Input: part model. Units: mm. Frame: model coordinates. A direction names the side the tool comes from. Coordinates: 2 decimals unless noted, no trailing zeros. Order: outer loops, then holes, each group sorted by start corner. A loop starts at its lowest first (then second) coordinate and runs counter-clockwise, first axis right, second up.
from build123d import *

# Parameters (mm, degrees)
SKETCH1_R           = 1.5
BOSS_EXTRUDE1_DEPTH = 10
BOSS_EXTRUDE2_DEPTH = 1.75
SKETCH3_R           = 3
CUT_EXTRUDE1_DEPTH  = 5


with BuildPart() as part:
    # Sketch1 → Boss-Extrude1 (new body)
    with BuildSketch(Plane(origin=(0, 0, 0), x_dir=(1, 0, 0), z_dir=(0, 1, 0))):
        with BuildLine():
            ThreePointArc((-43.97114317, 22.5), (-38.97114317, 17.5), (-33.97114317, 22.5))
            Line((-33.97114317, 22.5), (-33.97114317, 54.272052467))
            Line((-33.97114317, 54.272052467), (33.97114317, 54.272052467))
            Line((33.97114317, 54.272052467), (33.97114317, 22.5))
            ThreePointArc((33.97114317, 22.5), (38.97114317, 17.5), (43.97114317, 22.5))
            Line((43.97114317, 22.5), (43.97114317, 64.272052467))
            Line((43.97114317, 64.272052467), (-43.97114317, 64.272052467))
            Line((-43.97114317, 64.272052467), (-43.97114317, 22.5))
        make_face()
        with Locations(Location((-38.97114317, 22.5, 0), (0, 0, 270))):
            Circle(SKETCH1_R, mode=Mode.SUBTRACT)
        with Locations(Location((38.97114317, 22.5, 0), (0, 0, 270))):
            Circle(SKETCH1_R, mode=Mode.SUBTRACT)
        with Locations(Location((7.5, 59.272052467, 0), (0, 0, 270))):
            Circle(SKETCH1_R, mode=Mode.SUBTRACT)
        with Locations(Location((-7.5, 59.272052467, 0), (0, 0, 270))):
            Circle(SKETCH1_R, mode=Mode.SUBTRACT)
    extrude(amount=BOSS_EXTRUDE1_DEPTH)

    # Sketch2 → Boss-Extrude2 (add)
    # profile 1 of 2: a face of its own
    with BuildSketch(Plane.XZ):
        Polygon((-1.726497308, -59.272052467), (-4.613248654, -54.272052467), (-10.386751346, -54.272052467), (-13.273502692, -59.272052467), (-10.386751346, -64.272052467), (-4.613248654, -64.272052467), align=None)
        Polygon((-9.232050808, -56.272052467), (-5.767949192, -56.272052467), (-4.035898385, -59.272052467), (-5.767949192, -62.272052467), (-9.232050808, -62.272052467), (-10.964101615, -59.272052467), align=None, mode=Mode.SUBTRACT)
    # profile 2 of 2: a face of its own
    with BuildSketch(Plane.XZ):
        Polygon((10.386751346, -54.272052467), (4.613248654, -54.272052467), (1.726497308, -59.272052467), (4.613248654, -64.272052467), (10.386751346, -64.272052467), (13.273502692, -59.272052467), align=None)
        Polygon((5.767949192, -56.272052467), (9.232050808, -56.272052467), (10.964101615, -59.272052467), (9.232050808, -62.272052467), (5.767949192, -62.272052467), (4.035898385, -59.272052467), align=None, mode=Mode.SUBTRACT)
    extrude(amount=BOSS_EXTRUDE2_DEPTH)

    # Sketch3 → Cut-Extrude1 (cut)
    with BuildSketch(Plane(origin=(0, 10, 0), x_dir=(1, 0, 0), z_dir=(0, 1, 0))):
        with Locations(Location((-38.97114317, 22.5, 0), (0, 0, 270))):
            Circle(SKETCH3_R)
        with Locations(Location((38.97114317, 22.5, 0), (0, 0, 270))):
            Circle(SKETCH3_R)
    extrude(amount=-CUT_EXTRUDE1_DEPTH, mode=Mode.SUBTRACT)


solid = part.part
Item 1: Cut plane D-D on x = 17. Return loops of the section in (y, z).
Response values:
outline: (0, -64.27) - (10, -64.27) - (10, -54.27) - (0, -54.27) - close
Item 2: Cut plane C-C on y = 1.75. Return loops of the section in (x, z), then the cut area to 3 significant figures.
Response values:
outline: (-43.97, -64.27) - (43.97, -64.27) - (43.97, -22.5) arc R5 ccw to (33.97, -22.5) - (33.97, -54.27) - (-33.97, -54.27) - (-33.97, -22.5) arc R5 ccw to (-43.97, -22.5) - close; hole circle Ø3 at (-38.97, -22.5); hole circle Ø3 at (-7.5, -59.27); hole circle Ø3 at (7.5, -59.27); hole circle Ø3 at (38.97, -22.5)
area: 1,570 mm2
Item 3: Pin query (flat end, axial travel): pin 1 Ø17 at (x, z) = (-29.5, -48) entering from -Y; pin 2 Ø4 at (x, z) = (-0.5, -58.5) entering from -Y; pin 3 Ø0.9 at (x, y) = (-7, -1) entering from +Z; pin 4 Ø5 at (x, z) = (38.97, -22.5) entering from +Y. Return the tip coordinate at first contact, or that it passes through.
Response values:
pin 1: stops at y = 0
pin 2: stops at y = -1.75
pin 3: stops at z = -54.27
pin 4: stops at y = 5
Item 4: Draft query along X for faces 1 (the face through (8, 0, -61)), 2 (the face through (-11.81, -0.86, -56.74)), 3 (the face through (11.81, -0.86, -61.81)). Return one class per face: pulls with the +X half, pulls with the -X half, needs draft (parallel to the pull), parting line crosses it, or undercut.
Response values:
face 1: undercut
face 2: pulls with the -X half
face 3: pulls with the +X half
Item 5: Access query for faces 4 (the face through (-11.85, -0.86, -61.74)), 5 (the face through (-3.15, -0.86, -56.81)), 6 (the face through (11.85, -0.86, -56.81)), 7 (the face through (38, 5, -24)), 8 (the face through (3.15, -0.86, -61.74)). Directions: +Z, -Z, +X, -X, +Y, -Y. A direction counts if a zero-diameter tool reaches every point of the face in a straight line with its end or side. Return the directions, or none.
Response values:
face 4: -Z, -X, -Y
face 5: +Z, -Y
face 6: +Z, +X, -Y
face 7: +Y
face 8: -Z, -Y
Item 6: Cut plane A-A on z = -30. Return loops of the section in (x, y), then the cut area to 3 significant figures.
Response values:
outline: (-43.97, 0) - (-33.97, 0) - (-33.97, 10) - (-43.97, 10) - close; (33.97, 0) - (43.97, 0) - (43.97, 10) - (33.97, 10) - close
area: 200 mm2
Item 7: Ray query, probe 1 along X at (y, z) = (7.4, -22.5); probe 2 along X at (y, z) = (6, -32.5); probe 3 along X at (y, z) = (1.25, -23.5). Return the intervals inside material, ascending.
Response values:
probe 1: x = -43.97 to -41.97, -35.97 to -33.97, 33.97 to 35.97, 41.97 to 43.97
probe 2: x = -43.97 to -33.97, 33.97 to 43.97
probe 3: x = -43.97 to -40.09, -37.85 to -33.97, 33.97 to 37.85, 40.09 to 43.97
Item 8: Cut plane B-B on x = -7.5. Return loops of the section in (y, z).
Response values:
outline: (-1.75, -64.27) - (10, -64.27) - (10, -60.77) - (0, -60.77) - (0, -62.27) - (-1.75, -62.27) - close; (-1.75, -56.27) - (0, -56.27) - (0, -57.77) - (10, -57.77) - (10, -54.27) - (-1.75, -54.27) - close
